Could you check a few things on this model? Use its own coordinates, in mm. A direction names the side the tool comes from. Round coordinates to 2 decimals unless told otherwise and drop trailing zeros. Write each loop counter-clockwise with the first axis right and the second up, starting at its lowest first coordinate (ties: lowest second). Pieces come first, ordered by that corner, then holes. Notation, with made-up numbers: M 77.25,75 L 131.25,75 A28 cw 131.25,98 Z; hole C -32.75,-23.5 d8. An arc over 180 degrees is marked long. One line per item, written item: value. Start each with the question number.
(1) If I drill on L1, parallel to X at y = -1.4, z = 81; L2, parallel to Z at x = 11, y = -5.15; L3, parallel to Z at x = -11, y = -4.05, over which ranges is the centre line in solid material (lowest first)?
(2) I want a section at A-A on y = -4.95. Please give me the cut outline in (x, z), and give its area (3 significant figures).
(3) I'm going to push flat-ended pins straight in: pin 1 Ø2 at (x, z) = (4.5, 55) entering from +Y; pin 2 Ø2 at (x, y) = (4, -3.5) entering from +Z; pin 3 Ø1 at (x, y) = (6.5, -4) entering from +Z; pin 4 Ø3 at (y, z) = (-3.5, 33.5) entering from -X. Where does each tip first touch, or does it pass through?
(4) Thinking about a two-plate mould opening in Z: for faces 1 (the face through (-8.757, -2.958, 74.501)), 2 (the face through (4.488, -2.958, 78.744)), 3 (the face through (-3, -3, 32)), which applies, released by +Z, released by -Z, zero draft, split by the parting line, or undercut?
(5) I want a section at B-B on x = -7.75. Please give me the cut outline in (y, z), and give its area (3 significant figures).
(6) I want a section at C-C on z = 44. Please give me the cut outline in (x, y), and give its area (3 significant figures).
(7) Which directions (+Z, -Z, +X, -X, +Y, -Y) give clear straight access to the entire face, cutting with the end or side of a thin tool? Please do faces 4 (the face through (-4.39, -2.96, 78.62)), 5 (the face through (5.892, -2.958, 59.853)), 6 (the face through (-8.633, -2.958, 65.623)), 7 (the face through (-13.181, -2.958, 56.926)), 8 (the face through (8.73, -2.96, 65.5)).
```python
from build123d import *

# Parameters (mm, degrees)
F0_R     = 0.5
F1_DEPTH = 6


with BuildPart() as f1:
    # F0 (on Front) → F1 (new body)
    with BuildSketch(Plane.XZ):
        with BuildLine():
            Line((-3, 62.770455), (-3, 0))
            Line((-3, 0), (3, 0))
            Line((3, 0), (3, 62.744264))
            Line((3, 62.744264), (8.865584, 56.87868))
            ThreePointArc((8.865584, 56.87868), (13.108225, 56.87868), (13.108225, 61.12132))
            Line((13.108225, 61.12132), (4.229545, 70))
            Line((4.229545, 70), (13.108225, 78.87868))
            ThreePointArc((13.108225, 78.87868), (13.108225, 83.12132), (8.865584, 83.12132))
            Line((8.865584, 83.12132), (-0.013096, 74.242641))
            Line((-0.013096, 74.242641), (-8.891775, 83.12132))
            ThreePointArc((-8.891775, 83.12132), (-13.134416, 83.12132), (-13.134416, 78.87868))
            Line((-13.134416, 78.87868), (-4.255736, 70))
            Line((-4.255736, 70), (-13.134416, 61.12132))
            ThreePointArc((-13.134416, 61.12132), (-13.134416, 56.87868), (-8.891775, 56.87868))
            Line((-8.891775, 56.87868), (-3, 62.770455))
        make_face()
        with Locations((-11.013096, 59)):
            Circle(F0_R, mode=Mode.SUBTRACT)
        with Locations((-11.013096, 81)):
            Circle(F0_R, mode=Mode.SUBTRACT)
        with Locations((10.986904, 59)):
            Circle(F0_R, mode=Mode.SUBTRACT)
        with Locations((10.986904, 81)):
            Circle(F0_R, mode=Mode.SUBTRACT)
    extrude(amount=F1_DEPTH)


solid = f1.part
```
Found:
1. L1: x = -14.01 to -11.51, -10.51 to -6.77, 6.74 to 10.49, 11.49 to 13.99
1. L2: z = 56 to 58.5, 59.5 to 63.23, 76.77 to 80.5, 81.5 to 84
1. L3: z = 56 to 58.5, 59.5 to 63.26, 76.74 to 80.5, 81.5 to 84
2. outline: M -13.13,61.12 A3 ccw -8.89,56.88 L -3,62.77 L -3,0 L 3,0 L 3,62.74 L 8.87,56.88 A3 ccw 13.11,61.12 L 4.23,70 L 13.11,78.88 A3 ccw 8.87,83.12 L -0.01,74.24 L -8.89,83.12 A3 ccw -13.13,78.88 L -4.26,70 Z; hole C -11.01,59 d1; hole C -11.01,81 d1; hole C 10.99,59 d1; hole C 10.99,81 d1
2. area: 776 mm²
3. pin 1: passes through
3. pin 2: stops at z = 79.26
3. pin 3: stops at z = 81.26
3. pin 4: stops at x = -3
4. face 1: undercut
4. face 2: released by +Z
4. face 3: zero draft
5. outline: M -6,58.02 L 0,58.02 L 0,66.51 L -6,66.51 Z; M -6,73.49 L 0,73.49 L 0,81.98 L -6,81.98 Z
5. area: 102 mm²
6. outline: M -3,-6 L 3,-6 L 3,0 L -3,0 Z
6. area: 36.0 mm²
7. face 4: +Z, +Y, -Y
7. face 5: -Z, +Y, -Y
7. face 6: -X, +Y, -Y
7. face 7: +Y, -Y
7. face 8: +X, +Y, -Y
